from build123d import *

# Parameters (mm, degrees)
SKETCH_W        = 9
SKETCH_H        = 9
PAD_DEPTH       = 1.8
SKETCH001_R     = 0.25
POCKET_DEPTH    = 0.25
SKETCH002_W     = 3.2
SKETCH002_H     = 0.6
POCKET001_DEPTH = 1


with BuildPart() as part:
    # Sketch → Pad (new body)
    with BuildSketch(Plane.XY):
        Rectangle(SKETCH_W, SKETCH_H)
    extrude(amount=PAD_DEPTH)

    # Sketch001 (on Face6 of Pad) → Pocket (cut)
    with BuildSketch(Plane.XY.offset(1.8)):
        with Locations((3, 3)):
            Circle(SKETCH001_R)
    extrude(amount=-POCKET_DEPTH, mode=Mode.SUBTRACT)

    # Sketch002 (on Face6 of Pocket) → Pocket001 (cut)
    with BuildSketch(Plane.YZ.offset(4.5)):
        with Locations((0, 0.3)):
            Rectangle(SKETCH002_W, SKETCH002_H)
    pocket001 = extrude(amount=-POCKET001_DEPTH, mode=Mode.SUBTRACT)

    # Mirrored: Pocket001 across YZ
    add(pocket001.mirror(Plane.YZ), mode=Mode.SUBTRACT)


solid = part.part
For this review, take the finished solid that the model builds, in its own axes (mm). Round coordinates to 2 decimals unless told otherwise and drop trailing zeros. Loops run counter-clockwise (first coordinate to the right, second up) from the corner with the lowest first, then second, coordinate; pieces in that order, holes last. Notation, with made-up numbers: (22, 17) - (35, 17) arc R22 ccw to (35, 26) - close; hole circle Ø5 at (-34, 65.25). An arc over 180 degrees is marked (long way). Use one line per item in the form item = value.
1) We need section A-A on z = 0.35. Write out the cut boundary in (x, y).
Solutions:
outline = (-4.5, -4.5) - (4.5, -4.5) - (4.5, -1.6) - (3.5, -1.6) - (3.5, 1.6) - (4.5, 1.6) - (4.5, 4.5) - (-4.5, 4.5) - (-4.5, 1.6) - (-3.5, 1.6) - (-3.5, -1.6) - (-4.5, -1.6) - close
2) Mouldability with a two-part tool opening along Y and no side actions: class faces 1 (the face through (-4.5, 0, 1)), 2 (the face through (0, -4.5, 1)), 3 (the face through (-4, 0, 0.6)), 4 (the face through (4, 0, 0.6)) as pulls with the +Y half, pulls with the -Y half, needs draft (parallel to the pull), parting line crosses it, or undercut.
Solutions:
face_1 = needs draft
face_2 = pulls with the -Y half
face_3 = undercut
face_4 = undercut
3) We need section B-B on x = 3.75. Write out the cut boundary in (y, z), then the cut area to 3 significant figures.
Solutions:
outline = (-4.5, 0) - (-1.6, 0) - (-1.6, 0.6) - (1.6, 0.6) - (1.6, 0) - (4.5, 0) - (4.5, 1.8) - (-4.5, 1.8) - close
area = 14.3 mm2
4) Wall thickness on probe 1 along Y at (x, z) = (3, 1.7); probe 2 along Y at (x, z) = (4, 0.3): over which ranges is each line inside the solid? List them lowest first.
Solutions:
probe_1 = -4.5 to 2.75, 3.25 to 4.5
probe_2 = -4.5 to -1.6, 1.6 to 4.5
5) Clearance check with flat-ended pins moving along their axes: P1, Ø0.5, axis at x = -4, y = 0, coming from the -Z side; P2, Ø0.7, axis at y = -0.5, z = 0, coming from the +X side. State where each tip first meets the part, or that it passes through.
Solutions:
P1 = 0.6
P2 = 3.5
